Source: CAD feature listing. Evaluate the final solid. Frame: model axes, mm. Face numbers are marked on the shaded views. A direction names the side the tool comes from. Round coordinates to 2 decimals unless told otherwise and drop trailing zeros. Write each loop counter-clockwise with the first axis right and the second up, starting at its lowest first coordinate (ties: lowest second). Pieces come first, ordered by that corner, then holes. Notation, with made-up numbers: M -12.75,42 L 34.25,42 A22 cw 34.25,57 Z; hole C 60,-29.5 d1. An arc over 180 degrees is marked long. Answer in a Markdown table with one row per item. Add a question column.
Item 1: Mould query, pull axis Y, two halves, no side actions, for the marked faces 1, 2 and 3. Classes: released by +Y, released by -Y, zero draft, split by the parting line, or undercut.
Item 2: Cut plane B-B on z = 126.5. Return loops of the section in (x, y), and give its area (3 significant figures).
Item 3: Set-up query: the marked faces 4 and 5. Return all of +Z, -Z, +X, -X, +Y, -Y with unobstructed straight access to the full face (end or side cutting, diameter ignored); none if empty.
Item 4: Cut plane C-C on y = 0. Return loops of the section in (x, z).
Item 5: Cut plane A-A on x = -36. Return loops of the section in (y, z).
Item 6: Material intervals for probe 1 along Y at (x, z) = (-25, 171); probe 2 along X at (y, z) = (15, 126); probe 3 along X at (y, z) = (-4, 101), sorted ascending.
Item 7: Contact query for flat-ended pins moving along their axis: pin 1 (12 mm diameter, centred on y = -14.5, z = 20.5, fed in from +X); pin 2 (0.6 mm diameter, centred on y = 18, z = 51.5, fed in from -X); pin 3 (25 mm diameter, centred on x = -24.5, z = 90.5, fed in from +Y). Output: stop coordinate, or through.
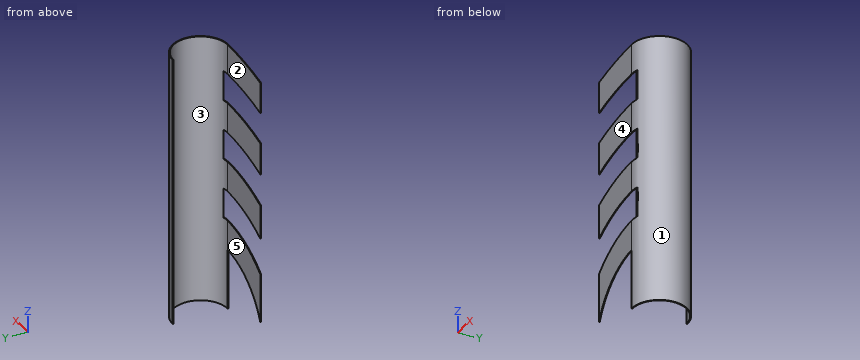
from build123d import *

# Parameters (mm, degrees)
SKETCH_1_R           = 18.5
SKETCH_1_R_2         = 18
EXTRUDE_1_DEPTH      = 180
SKETCH_15_W          = 19.647344242
SKETCH_15_H          = 48.423013506
CUT_EXTRUDE_7_DEPTH  = 208.5
SKETCH_16_W          = 20
SKETCH_16_H          = 0.5
EXTRUDE_4_DEPTH      = 40
SKETCH_17_W          = 20
SKETCH_17_H          = 1
CUT_EXTRUDE_8_DEPTH  = 40
EXTRUDE_8_DEPTH      = 0.5
CUT_EXTRUDE_10_DEPTH = 0.5


with BuildPart() as part:
    # 草图1 → 凸台-拉伸1 (new body)
    with BuildSketch(Plane.XY):
        with Locations(Location((0, 0, 0), (0, 0, 180))):
            Circle(SKETCH_1_R)
        with Locations(Location((0, 0, 0), (0, 0, 180))):
            Circle(SKETCH_1_R_2, mode=Mode.SUBTRACT)
    extrude(amount=EXTRUDE_1_DEPTH)

    # 草图15 → 切除-拉伸7 (cut, symmetric)
    with BuildSketch(Plane(origin=(0, 0, 0), x_dir=(-1, 0, 0), z_dir=(0, 0, -1))):
        with Locations((9.823672121, -2.226084919)):
            Rectangle(SKETCH_15_W, SKETCH_15_H)
    extrude(amount=CUT_EXTRUDE_7_DEPTH, both=True, mode=Mode.SUBTRACT)

    # 草图16 → 凸台-拉伸4 (add)
    with BuildSketch(Plane(origin=(0, 0, 0), x_dir=(0, 0, -1), z_dir=(1, 0, 0))):
        with Locations((-90, -18.25)):
            Rectangle(SKETCH_16_W, SKETCH_16_H)
        with Locations((-50, -18.25)):
            Rectangle(SKETCH_16_W, SKETCH_16_H)
        with Locations((-130, -18.25)):
            Rectangle(SKETCH_16_W, SKETCH_16_H)
        with Locations((-170, -18.25)):
            Rectangle(SKETCH_16_W, SKETCH_16_H)
    extrude(amount=-EXTRUDE_4_DEPTH)

    # 草图17 → 切除-拉伸8 (cut)
    with BuildSketch(Plane(origin=(0, 0, 0), x_dir=(0, 0, -1), z_dir=(1, 0, 0))):
        with Locations((-110, -18)):
            Rectangle(SKETCH_17_W, SKETCH_17_H)
        with Locations((-150, -18)):
            Rectangle(SKETCH_17_W, SKETCH_17_H)
        with Locations((-70, -18)):
            Rectangle(SKETCH_17_W, SKETCH_17_H)
    extrude(amount=CUT_EXTRUDE_8_DEPTH, mode=Mode.SUBTRACT)

    # 草图20 → 凸台-拉伸8 (add)
    with BuildSketch(Plane.XZ.offset(18.5)):
        with BuildLine():
            Line((0, 59.952777719), (0, 39.932309719))
            ThreePointArc((0, 39.932309719), (-24.004305164, 31.641271223), (-40, 11.916015014))
            Line((-40, 11.916015014), (-40, 44.556181889))
            ThreePointArc((-40, 44.556181889), (-21.280533863, 55.581277174), (0, 59.952777719))
        make_face()
        with BuildLine():
            Line((-40, 68.814162833), (-40, 91.125176599))
            ThreePointArc((-40, 91.125176599), (-20.430552708, 97.494887784), (0, 99.97057031))
            Line((0, 99.97057031), (0, 79.980767144))
            ThreePointArc((0, 79.980767144), (-20.682391226, 76.84186512), (-40, 68.814162833))
        make_face()
        with BuildLine():
            Line((0, 180), (0, 159.99002565))
            ThreePointArc((0, 159.99002565), (-20.167840481, 158.455833888), (-40, 154.483305373))
            Line((-40, 154.483305373), (-40, 175.102068383))
            ThreePointArc((-40, 175.102068383), (-20.132883898, 178.636258798), (0, 180))
        make_face()
        with BuildLine():
            Line((-40, 112.628405695), (-40, 133.686346725))
            ThreePointArc((-40, 133.686346725), (-20.218894936, 138.224000128), (0, 139.978623608))
            Line((0, 139.978623608), (0, 119.975235288))
            ThreePointArc((0, 119.975235288), (-20.297894119, 117.923712576), (-40, 112.628405695))
        make_face()
    extrude(amount=-EXTRUDE_8_DEPTH)

    # 草图21 → 切除-拉伸10 (cut)
    with BuildSketch(Plane.XZ.offset(18.5)):
        with BuildLine():
            Line((0, 79.980767144), (0, 59.952777719))
            ThreePointArc((0, 59.952777719), (-21.280533863, 55.581277174), (-40, 44.556181889))
            Line((-40, 44.556181889), (-40, 68.814162833))
            ThreePointArc((-40, 68.814162833), (-20.682391226, 76.84186512), (0, 79.980767144))
        make_face()
        with BuildLine():
            Line((-40, 91.405123559), (-40, 112.628405695))
            ThreePointArc((-40, 112.628405695), (-20.297894119, 117.923712576), (0, 119.975235288))
            Line((0, 119.975235288), (0, 100.22725283))
            ThreePointArc((0, 100.22725283), (-20.428312001, 97.758177426), (-40, 91.405123559))
        make_face()
        with BuildLine():
            Line((0, 159.99002565), (0, 140.07912782))
            ThreePointArc((0, 140.07912782), (-20.218582252, 138.325773675), (-40, 133.791368433))
            Line((-40, 133.791368433), (-40, 154.483305373))
            ThreePointArc((-40, 154.483305373), (-20.167840481, 158.455833888), (0, 159.99002565))
        make_face()
        with BuildLine():
            Line((-40, 175.084831136), (-40, 180))
            Line((-40, 180), (-40, 184.582306451))
            Line((-40, 184.582306451), (-35.32938599, 184.045292069))
            Line((-35.32938599, 184.045292069), (0, 179.983216215))
            ThreePointArc((0, 179.983216215), (-20.132908432, 178.619348164), (-40, 175.084831136))
        make_face()
    extrude(amount=-CUT_EXTRUDE_10_DEPTH, mode=Mode.SUBTRACT)


solid = part.part
Results below:
| question | item | result |
|---|---|---|
| 1 | face 1 | split by the parting line |
| 1 | face 2 | released by +Y |
| 1 | face 3 | undercut |
| 2 | outline | M -40,-18.5 L 0,-18.5 A18.5 ccw 0,18.5 L 0,18 A18 cw 0,-18 L -40,-18 Z |
| 2 | area | 48.7 mm2 |
| 3 | face 4 | +Z, -Z, +X, -X, -Y |
| 3 | face 5 | +Z, -Z, -X, +Y |
| 4 | outline | M 18,0 L 18.5,0 L 18.5,180 L 18,180 Z |
| 5 | outline | M -18.5,19.34 L -18,19.34 L -18,47.65 L -18.5,47.65 Z; M -18.5,70.94 L -18,70.94 L -18,93.05 L -18.5,93.05 Z; M -18.5,113.98 L -18,113.98 L -18,134.94 L -18.5,134.94 Z; M -18.5,155.49 L -18,155.49 L -18,175.98 L -18.5,175.98 Z |
| 6 | probe 1 | -18.5 to -18 |
| 6 | probe 2 | 9.95 to 10.83 |
| 6 | probe 3 | 17.55 to 18.06 |
| 7 | pin 1 | x = 16.43 |
| 7 | pin 2 | x = 0 |
| 7 | pin 3 | y = -18 |
